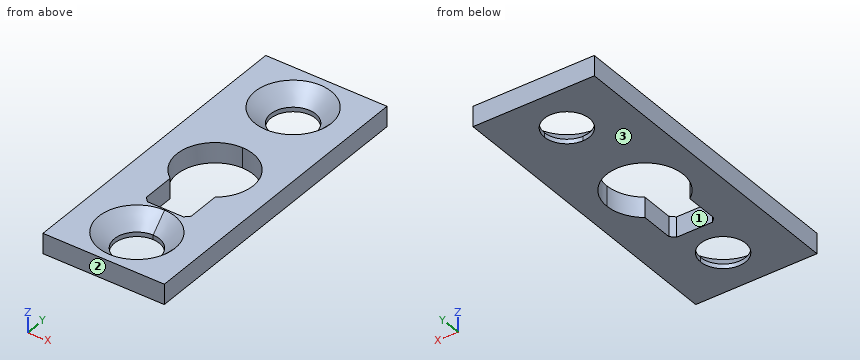
```python
from build123d import *

# Parameters (mm, degrees)
F0_W     = 13.5
F0_H     = 34.2
F1_DEPTH = 2.25
F2_SIZE  = 0.5
F3_SIZE  = 1.75


with BuildPart() as f1:
    # F0 (on Top) → F1 (new body)
    with BuildSketch(Plane.XY):
        Rectangle(F0_W, F0_H)
        with BuildLine():
            ThreePointArc((2.5, -12), (-1.767766953, -13.767766953), (0, -9.5))
            ThreePointArc((0, -9.5), (1.767766953, -10.232233047), (2.5, -12))
        make_face(mode=Mode.SUBTRACT)
        with BuildLine():
            ThreePointArc((-2.5, -3.4369317712), (-4.041624675, 1.3144466464), (0, 4.25))
            ThreePointArc((0, 4.25), (3.00520382, 3.00520382), (4.25, 0))
            ThreePointArc((4.25, 0), (3.7873143519, -1.9284060776), (2.5, -3.4369317712))
            Line((2.5, -3.4369317712), (2.5, -7.6))
            Line((2.5, -7.6), (0, -7.6))
            Line((0, -7.6), (-2.5, -7.6))
            Line((-2.5, -7.6), (-2.5, -3.4369317712))
        make_face(mode=Mode.SUBTRACT)
        with BuildLine():
            ThreePointArc((2.5, 12), (1.767766953, 10.232233047), (0, 9.5))
            ThreePointArc((0, 9.5), (-1.767766953, 13.767766953), (2.5, 12))
        make_face(mode=Mode.SUBTRACT)
    extrude(amount=F1_DEPTH)

    # F2
    f2_edges = [f1.edges().sort_by_distance(p)[0] for p in [
        (-2.5, -7.6, 1.125),
        (2.5, -7.6, 1.125),
    ]]
    chamfer(f2_edges, length=F2_SIZE)

    # F3
    f3_edges = [f1.edges().sort_by_distance(p)[0] for p in [
        (0, -14.5, 2.25),
        (-2.5, 12, 2.25),
    ]]
    chamfer(f3_edges, length=F3_SIZE)


solid = f1.part
```
Design review of the part built by this model. Coordinates are the model's own, in mm. Face numbers are marked on the shaded views. Coordinates: 2 decimals unless noted, no trailing zeros. Order: outer loops, then holes, each group sorted by start corner. A loop starts at its lowest first (then second) coordinate and runs counter-clockwise, first axis right, second up. Notation, with made-up numbers: M 20,-37.5 L 35,-37.5 A12 cw 35,-17.5 Z; hole C 65.25,54 d1. An arc over 180 degrees is marked long. Answer as a JSON object with one key per item and string values. Group by question number.
1) Mouldability with a two-part tool opening along Y and no side actions: class the marked faces 1, 2 and 3 as pulls with the +Y half, pulls with the -Y half, needs draft (parallel to the pull), parting line crosses it, or undercut.
2) Add section B-B, the plane y = 2. Write out the cut boundary in (x, z), then the cut area to 3 significant figures.
3) Add section C-C, the plane y = -6.5. Write out the cut boundary in (x, z).
4) Add section D-D, the plane x = -1.25. Count the separate pieces of the cut face and the enclosed holes in it, then the cut area to 3 significant figures.
5) Wall thickness on L1, parallel to Y at x = -0.5, z = 0.4; L2, parallel to X at y = 12, z = 0.1; L3, parallel to Y at x = -2.25, z = 2: over which ranges is each line inside the solid? List them lowest first.
6) For pin 1 (4.5 mm diameter, centred on x = 0, y = 12, fed in from +Z), flat-tipped, find the tip position at first contact; note if it passes through.
7) Add section A-A, the plane z = 0.8. Write out the cut boundary in (x, y).
Computed values:
{
 "1": {"face 1": "undercut", "face 2": "pulls with the -Y half", "face 3": "needs draft"},
 "2": {"outline": "M -6.75,0 L -3.75,0 L -3.75,2.25 L -6.75,2.25 Z; M 3.75,0 L 6.75,0 L 6.75,2.25 L 3.75,2.25 Z", "area": "13.5 mm^2"},
 "3": {"outline": "M -6.75,0 L -2.5,0 L -2.5,2.25 L -6.75,2.25 Z; M 2.5,0 L 6.75,0 L 6.75,2.25 L 2.5,2.25 Z"},
 "4": {"separate pieces": "4", "enclosed holes": "0", "area": "24.5 mm^2"},
 "5": {"L1": "y = -17.1 to -14.45, -9.55 to -7.6, 4.22 to 9.55, 14.45 to 17.1", "L2": "x = -6.75 to -2.5, 2.5 to 6.75", "L3": "y = -17.1 to -15.31, -8.69 to -7.35, 3.61 to 8.69, 15.31 to 17.1"},
 "6": {"pin 1": "passes through"},
 "7": {"outline": "M -6.75,-17.1 L 6.75,-17.1 L 6.75,17.1 L -6.75,17.1 Z; hole C 0,-12 d5.6; hole C 0,12 d5.6; hole M -2.5,-7.1 L -2,-7.6 L 2,-7.6 L 2.5,-7.1 L 2.5,-3.44 A4.25 ccw long -2.5,-3.44 Z"}
}
